Input: part model. Units: mm. Frame: model coordinates. A direction names the side the tool comes from. Give positions to 0.01 mm unless a question says otherwise; leave off trailing zeros. Write each loop counter-clockwise with the first axis right and the second up, starting at its lowest first coordinate (ties: lowest second). Pieces come first, ordered by that corner, then holes.
```python
from build123d import *

# Parameters (mm, degrees)
F1_DEPTH  = 12.5
F2_R      = 6
F3_DEPTH  = 25
F4_R      = 13
F5_DEPTH  = 20
F6_W      = 32
F6_H      = 32
F7_DEPTH  = 5
F8_R      = 7
F9_DEPTH  = 5
F10_SIZE  = 5
F11_SIZE  = 5
F12_R     = 2.75
F13_DEPTH = 25
F14_SIZE  = 2


with BuildPart() as f1:
    # F0 (on Front) → F1 (new body, symmetric)
    with BuildSketch(Plane.XZ):
        Polygon((17, 11), (17, 21.5), (-17, 21.5), (-17, 11), (-30, 11), (-30, -21.5), (30, -21.5), (30, 11), align=None)
    extrude(amount=F1_DEPTH, both=True)

    # F2 (on face) → F3 (cut)
    with BuildSketch(Plane.XZ.offset(12.5)):
        with Locations((0, 3.5)):
            Circle(F2_R)
    extrude(amount=-F3_DEPTH, mode=Mode.SUBTRACT)

    # F4 (on face) → F5 (cut)
    with BuildSketch(Plane.XZ.offset(12.5)):
        with Locations((0, 3.5)):
            Circle(F4_R)
    extrude(amount=-F5_DEPTH, mode=Mode.SUBTRACT)

    # F6 (on face) → F7 (join)
    with BuildSketch(Plane.XZ.offset(12.5)):
        with Locations((0, 3.5)):
            Rectangle(F6_W, F6_H)
    extrude(amount=F7_DEPTH)

    # F8 (on face) → F9 (cut)
    with BuildSketch(Plane.XZ.offset(17.5)):
        with Locations((0, 3.5)):
            Circle(F8_R)
    extrude(amount=-F9_DEPTH, mode=Mode.SUBTRACT)

    # F10
    f10_edges = [f1.edges().sort_by_distance(p)[0] for p in [
        (-16, -15, 19.5),
        (-16, -15, -12.5),
        (16, -15, 19.5),
        (16, -15, -12.5),
    ]]
    chamfer(f10_edges, length=F10_SIZE)

    # F11
    f11_edges = [f1.edges().sort_by_distance(p)[0] for p in [
        (17, 0, 21.5),
        (-17, 0, 21.5),
    ]]
    chamfer(f11_edges, length=F11_SIZE)

    # F12 (on face) → F13 (cut)
    with BuildSketch(Plane(origin=(0, 12.5, 0), x_dir=(-1, 0, 0), z_dir=(0, 1, 0))):
        with Locations((-23, 3.5)):
            Circle(F12_R)
        with Locations((23, 3.5)):
            Circle(F12_R)
        with Locations((23, -14.5)):
            Circle(F12_R)
        with Locations((-23, -14.5)):
            Circle(F12_R)
    extrude(amount=-F13_DEPTH, mode=Mode.SUBTRACT)

    # F14
    f14_edges = [f1.edges().sort_by_distance(p)[0] for p in [
        (30, 0, 11),
        (-30, 0, 11),
    ]]
    chamfer(f14_edges, length=F14_SIZE)


solid = f1.part
```
Item 1: Section C-C (z = -14.5). Return loops of the section in (x, y).
Item 2: Section B-B (x = 0). Return loops of the section in (y, z).
Item 3: Mould query, pull axis X, two halves, no side actions, for faces 1 (the flat face through (-16, -15, 3)), 2 (the cylindrical face through (-20.253, 0.175, 3.621)), 3 (the flat face through (16, -15, 3)). Classes: +X half, -X half, draft (parallel to the pull), parting line (faces both ways), or undercut.
Item 4: Ray query, line 1 (Z direction, x = -23, y = 3.5); line 2 (X direction, y = -10.5, z = -1.5); line 3 (Y direction, x = 3.5, z = 10.5). Return the intervals inside material, ascending.
Item 5: Pin query (flat end, axial travel): pin 1 (5 mm diameter, centred on y = 0.5, z = 12.5, fed in from +X); pin 2 (4 mm diameter, centred on x = 14.5, y = -9, fed in from +Z); pin 3 (12 mm diameter, centred on x = -20, z = -16.5, fed in from -Y); pin 4 (5 mm diameter, centred on x = 23, z = 3.5, fed in from +Y). Return the tip coordinate at first contact, or that it passes through.
Item 6: Section D-D (x = 23). Return loops of the section in (y, z).
Item 7: Set-up query: faces 4 (the flat face through (13.5, -15, -10)), 5 (the cylindrical face through (3.763, -15.035, 9.402)), 6 (the flat face through (0, -15, 19.5)), 7 (the flat face through (-17, 0, 14)), 8 (the flat face through (23, 0, 11)). Return all of +Z, -Z, +X, -X, +Y, -Y with unobstructed straight access to the full face (end or side cutting, diameter ignored); none if empty.
Item 8: Section A-A (y = -5.75). Return loops of the section in (x, z).
Solved:
1. outline: (-30, -12.5) - (-25.75, -12.5) - (-25.75, 12.5) - (-30, 12.5) - close; (-20.25, -12.5) - (20.25, -12.5) - (20.25, 12.5) - (-20.25, 12.5) - close; (25.75, -12.5) - (30, -12.5) - (30, 12.5) - (25.75, 12.5) - close
2. outline: (-17.5, -12.5) - (-12.5, -12.5) - (-12.5, -21.5) - (12.5, -21.5) - (12.5, -2.5) - (7.5, -2.5) - (7.5, -9.5) - (-12.5, -9.5) - (-12.5, -3.5) - (-17.5, -3.5) - close; (-17.5, 10.5) - (-12.5, 10.5) - (-12.5, 16.5) - (7.5, 16.5) - (7.5, 9.5) - (12.5, 9.5) - (12.5, 21.5) - (-12.5, 21.5) - (-12.5, 19.5) - (-17.5, 19.5) - close
3. face 1: -X half
3. face 2: undercut
3. face 3: +X half
4. line 1: z = -21.5 to -17.25, -11.75 to 0.75, 6.25 to 11
4. line 2: x = -30 to -12, 12 to 30
4. line 3: y = -17.5 to -12.5, 7.5 to 12.5
5. pin 1: stops at x = 29
5. pin 2: stops at z = 21
5. pin 3: stops at y = -12.5
5. pin 4: passes through
6. outline: (-12.5, -21.5) - (12.5, -21.5) - (12.5, -17.25) - (-12.5, -17.25) - close; (-12.5, -11.75) - (12.5, -11.75) - (12.5, 0.75) - (-12.5, 0.75) - close; (-12.5, 6.25) - (12.5, 6.25) - (12.5, 11) - (-12.5, 11) - close
7. face 4: -Z, +X, -Y
7. face 5: -Y
7. face 6: +Z, +X, -X, -Y
7. face 7: +Z, -X, +Y, -Y
7. face 8: +Z, +X, +Y, -Y
8. outline: (-30, -21.5) - (30, -21.5) - (30, 9) - (28, 11) - (17, 11) - (17, 16.5) - (12, 21.5) - (-12, 21.5) - (-17, 16.5) - (-17, 11) - (-28, 11) - (-30, 9) - close; hole circle Ø5.5 at (-23, -14.5); hole circle Ø5.5 at (-23, 3.5); hole circle Ø26 at (0, 3.5); hole circle Ø5.5 at (23, -14.5); hole circle Ø5.5 at (23, 3.5)
